Design review of the part built by this model. Coordinates are the model's own, in mm. Give positions to 0.01 mm unless a question says otherwise; leave off trailing zeros. Order: outer loops, then holes, each group sorted by start corner. A loop starts at its lowest first (then second) coordinate and runs counter-clockwise, first axis right, second up. Notation, with made-up numbers: (-14.75, 83.25) -> (20.25, 83.25) arc R29 ccw to (20.25, 109.25) -> close; hole circle Ø5 at (0.25, 69.5). An arc over 180 degrees is marked (long way). One line per item, written item: value.
from build123d import *

# Parameters (mm, degrees)
F0_W     = 31.707764
F0_H     = 54.837252
F1_DEPTH = 25
F2_SIZE  = 5
F3_R     = 5


with BuildPart() as f1:
    # F0 (on Top) → F1 (new body)
    with BuildSketch(Plane.XY):
        Rectangle(F0_W, F0_H)
    extrude(amount=F1_DEPTH)

    # F2
    f2_edges = [f1.edges().sort_by_distance(p)[0] for p in [
        (15.853882, 27.418626, 12.5),
        (-15.853882, 27.418626, 12.5),
    ]]
    chamfer(f2_edges, length=F2_SIZE)

    # F3
    f3_edges = [f1.edges().sort_by_distance(p)[0] for p in [
        (-15.853882, -27.418626, 12.5),
        (15.853882, -27.418626, 12.5),
    ]]
    fillet(f3_edges, radius=F3_R)


solid = f1.part
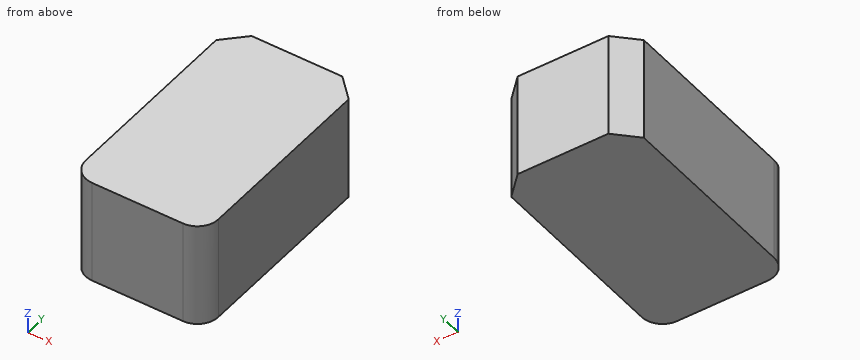
Item 1: Add section B-B on y = 23. Give the boundary of the cut face in (x, z).
Returned:
outline: (-15.27, 0) -> (15.27, 0) -> (15.27, 25) -> (-15.27, 25) -> close
Item 2: Add section C-C on x = 13. Give the boundary of the cut face in (y, z).
Returned:
outline: (-26.93, 0) -> (25.27, 0) -> (25.27, 25) -> (-26.93, 25) -> close
Item 3: To check wall thickness, follow line 1 along X through (y, z) = (-24.5, 3.75). State the ranges of the line that lie inside material, in increasing order. Write a range as from..to.
Returned:
line 1: -15.4..15.4
Item 4: Add section A-A on z = 6.5. Give the boundary of the cut face in (x, y), plus the area to 3 significant figures.
Returned:
outline: (-15.85, -22.42) arc R5 ccw to (-10.85, -27.42) -> (10.85, -27.42) arc R5 ccw to (15.85, -22.42) -> (15.85, 22.42) -> (10.85, 27.42) -> (-10.85, 27.42) -> (-15.85, 22.42) -> close
area: 1,700 mm²
